Input: part model. Units: mm. Frame: model coordinates. A direction names the side the tool comes from. Round coordinates to 2 decimals unless told otherwise and drop trailing zeros. Order: outer loops, then holes, each group sorted by start corner. A loop starts at its lowest first (then second) coordinate and runs counter-clockwise, first axis right, second up. Notation, with made-up numbers: M 52.25,-11 L 59.25,-11 A35 cw 59.25,25 Z; hole C 65.25,-4.5 d1. An arc over 180 degrees is marked long. One line per question, with ' | ' between items.
```python
from build123d import *


with BuildPart() as part:
    # Croquis1 → Revolución2 (revolve)
    with BuildSketch(Plane.XY):
        Polygon((8, 42.7), (4, 42.7), (4, 36.2), (2.1, 34.605710701), (2.1, 15.427573211), (3, 15.1), (3, 0), (11, 0), (11, 30), (8, 30), (8, 33), (6, 33), (6, 39), (8, 39), align=None)
    revolve(axis=Axis((0, 0, 0), (0, 1, 0)))

    # Croquis2 → Cortar-Revolución1 (revolve, cut)
    with BuildSketch(Plane.XY):
        Polygon((6.561668068, 0.7), (11, 0.7), (11, 1.7), (6.474179405, 1.7), align=None)
        Polygon((6.297452304, 3.72), (6.384940968, 2.72), (11, 2.72), (11, 3.72), align=None)
        Polygon((6.120725204, 5.74), (6.208213867, 4.74), (11, 4.74), (11, 5.74), align=None)
        Polygon((5.943998104, 7.76), (6.031486767, 6.76), (11, 6.76), (11, 7.76), align=None)
        Polygon((5.767271003, 9.78), (5.854759667, 8.78), (11, 8.78), (11, 9.78), align=None)
        Polygon((5.590543903, 11.8), (5.678032566, 10.8), (11, 10.8), (11, 11.8), align=None)
        Polygon((5.413816803, 13.82), (5.501305466, 12.82), (11, 12.82), (11, 13.82), align=None)
        Polygon((5.237089702, 15.84), (5.324578366, 14.84), (11, 14.84), (11, 15.84), align=None)
        Polygon((5.060362602, 17.86), (5.147851265, 16.86), (11, 16.86), (11, 17.86), align=None)
        Polygon((4.883635502, 19.88), (4.971124165, 18.88), (11, 18.88), (11, 19.88), align=None)
        Polygon((4.706908401, 21.9), (4.794397065, 20.9), (11, 20.9), (11, 21.9), align=None)
        Polygon((4.530181301, 23.92), (4.617669964, 22.92), (11, 22.92), (11, 23.92), align=None)
        Polygon((4.353454201, 25.94), (4.440942864, 24.94), (11, 24.94), (11, 25.94), align=None)
        Polygon((4.1767271, 27.96), (4.264215764, 26.96), (11, 26.96), (11, 29.98), (4, 29.98), (4.087488664, 28.98), (8, 28.98), (8, 27.96), align=None)
    revolve(axis=Axis((0, 0, 0), (0, 1, 0)), mode=Mode.SUBTRACT)

    # Croquis3 → Cortar-Revolución4 (revolve, cut)
    with BuildSketch(Plane.XY):
        Polygon((10.994525772, 30), (11.094314794, 30), (11.094314794, 29.98), (7.992627906, 29.98), (7.992627906, 30), align=None)
    revolve(axis=Axis((0, 0, 0), (0, 1, 0)), mode=Mode.SUBTRACT)


solid = part.part
```
Item 1: Section query B-B, the plane z = 7.5. Give the number of separate pieces and of enclosed holes in the cut face, plus the area to 3 significant figures.
Report:
separate pieces: 17 | enclosed holes: 0 | area: 268 mm²
Item 2: Mould query, pull axis Y, two halves, no side actions, for faces 1 (the flat face through (3.4, 27.96, 3.4)), 2 (the flat face through (-2.3, 0, 2.3)), 3 (the cylindrical face through (-2.38, 14.34, 10.74)). Classes: +Y half, -Y half, draft (parallel to the pull), parting line (faces both ways), or undercut.
Report:
face 1: undercut | face 2: -Y half | face 3: draft
Item 3: Line query: line 1 along Y through (x, z) = (4.5, 0); line 2 along Z through (x, y) = (0, 39.25); line 3 along Z through (x, y) = (0, 38.5). Output: solid intervals per line, ascending. Write a range as from..to.
Report:
line 1: 0..24.94, 25.94..26.96, 27.96..28.98, 29.98..42.7 | line 2: -8..-4, 4..8 | line 3: -6..-4, 4..6
Item 4: First-contact query: pin 1 (5 mm diameter, centred on y = 10.5, z = 5.5, fed in from -X); pin 2 (1 mm diameter, centred on y = 12, z = -1, fed in from -X); pin 3 (8 mm diameter, centred on x = 8.5, y = 14.5, fed in from -Z). Flat tips, straight axial feed; report the tip coordinate or a pass-through.
Report:
pin 1: x = -10.58 | pin 2: x = -10.99 | pin 3: z = -10.04
Item 5: Section query A-A, the plane y = 37. Return loops of the section in (x, z).
Report:
outline: C 0,0 d12; hole C 0,0 d8
Item 6: Access query for faces 4 (the cylindrical face through (-1.73, 40.88, 7.81)), 5 (the cylindrical face through (-2.38, 22.42, 10.74)), 6 (the flat face through (5, 7.76, 5)). Directions: +Z, -Z, +X, -X, +Y, -Y. A direction counts if a zero-diameter tool reaches every point of the face in a straight line with its end or side. Return the directions, or none.
Report:
face 4: +Y | face 5: +Y, -Y | face 6: none
